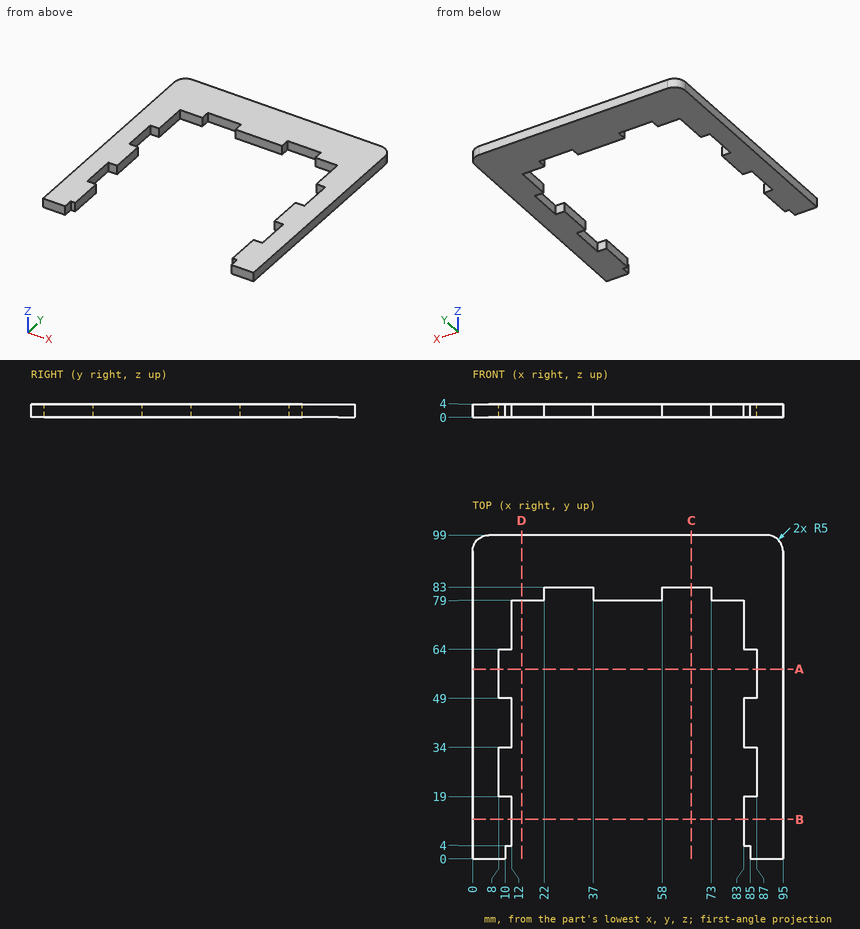
Study the drawing (mm; zero at the part's minimum x, y, z) and answer. Give positions to 0.01 mm unless a question says otherwise; leave off trailing zeros. Write each loop counter-clockwise with the first axis right and the second up, starting at its lowest first coordinate (ties: lowest second). Pieces come first, ordered by that corner, then holes. Notation, with made-up numbers: (13, -14.5) - (31, -14.5) arc R8 cw to (31, -10.5) - close; hole circle Ø1 at (18, 60). An arc over 180 degrees is marked (long way). Use a Markdown table: item, result.
1. Section C-C on x = 67 is taken. Write down the section's boundary in (y, z).
Values follow:
| item | result |
|---|---|
| outline | (83, 0) - (99, 0) - (99, 4) - (83, 4) - close |
2. Section A-A on y = 58 is taken. Write down the section's boundary in (x, z), plus the area to 3 significant figures.
Values follow:
| item | result |
|---|---|
| outline | (0, 0) - (8, 0) - (8, 4) - (0, 4) - close; (87, 0) - (95, 0) - (95, 4) - (87, 4) - close |
| area | 64.0 mm² |
3. This flat-tipped pin is pushed along its axis until it touches: P1, Ø0.6, axis at x = 83.5, z = 1, coming from the -Y side. Where does it stop, or does it pass through?
Values follow:
| item | result |
|---|---|
| P1 | stops at y = 4 |
4. Section D-D on x = 15 is taken. Write down the section's boundary in (y, z), plus the area to 3 significant figures.
Values follow:
| item | result |
|---|---|
| outline | (79, 0) - (99, 0) - (99, 4) - (79, 4) - close |
| area | 80.0 mm² |
5. Find the intervals of material crossed by probe 1 along X at (y, z) = (61, 2.55); probe 2 along X at (y, z) = (71, 3.6); probe 3 along Y at (x, z) = (23.5, 1.5), in increasing order. Write a range as from..to.
Values follow:
| item | result |
|---|---|
| probe 1 | x = 0..8, 87..95 |
| probe 2 | x = 0..12, 83..95 |
| probe 3 | y = 83..99 |
6. Section B-B on y = 12 is taken. Write down the section's boundary in (x, z), plus the area to 3 significant figures.
Values follow:
| item | result |
|---|---|
| outline | (0, 0) - (12, 0) - (12, 4) - (0, 4) - close; (83, 0) - (95, 0) - (95, 4) - (83, 4) - close |
| area | 96.0 mm² |
